Autodesk Inventor part; units mm, degrees
ref_plane "YZ Plane" through (0, 0, 0) normal (1, 0, 0) x (0, 1, 0)
ref_plane "XZ Plane" through (0, 0, 0) normal (0, 1, 0) x (-1, 0, 0)
ref_plane "XY Plane" through (0, 0, 0) normal (0, 0, 1) x (1, 0, 0)
sketch "Sketch1" plane through (0, 0, 0) normal (0, 0, 1) x (1, 0, 0)
  circle A0 centre (0, 0) radius 2.032
  circle A1 centre (0, 0) radius 5.08
  line L0 (3.81, 3.3601) -> (3.81, 5.5534)
  line L1 (-3.81, 3.3601) -> (-3.81, 6.2503)
  circle A2 centre (-20.9, 21.2222) radius 2.032
  circle A3 centre (-20.9, 21.2222) radius 5.08
  line L2 (-17.5399, 25.0322) -> (-14.2921, 25.0322)
  line L3 (-17.5399, 17.4122) -> (-14.7055, 17.4122)
  arc A4 (-3.81, 6.2503) -> (-14.7055, 17.4122) centre (-14.0813, 7.1228) ccw
  arc A5 (3.81, 5.5534) -> (-14.2921, 25.0322) centre (-14.2921, 6.8814) ccw
  point P0 (-3.81, 4.8052)
  dimension "d0" = 4.064
  dimension "d1" = 10.16
  dimension "d2" = 7.62
  dimension "d3" = 3.81
  dimension "d4" = 4.064
  dimension "d5" = 10.16
  dimension "d6" = 7.62
  dimension "d7" = 3.81
extrude "Extrusion1" add sketch "Sketch1" along normal blind 3.556
equation "\"d7\" = 0.5 * d6"
properties part number "Push Arm"
Source: CAD feature listing. Evaluate the final solid. Frame: model axes, mm. A direction names the side the tool comes from. Coordinates: 2 decimals unless noted, no trailing zeros. Loops run counter-clockwise (first coordinate to the right, second up) from the corner with the lowest first, then second, coordinate; pieces in that order, holes last. Notation, with made-up numbers: (-31, 38.5) -> (-7, 38.5) arc R17 cw to (-7, 44.5) -> close; hole circle Ø4 at (53.25, 64). An arc over 180 degrees is marked (long way). One line per item, written item: value. Start each with the question number.
Q1. Section query A-A, the plane y = 0. Return the cut outline in (x, z).
Q2. Contact query for flat-ended pins moving along their axis: P1, Ø2, axis at y = 5, z = 1.5, coming from the +X side; P2, Ø2, axis at y = 5.5, z = 3, coming from the -X side; P3, Ø0.9, axis at x = -17, z = 1.5, coming from the -Y side; P4, Ø2.5, axis at x = -20.9, y = 21.22, coming from the +Z side (3 decimals). Output: stop coordinate, or through.
Q3. Mould query, pull axis Y, two halves, no side actions, for faces 1 (the face through (-3.81, 5, 2)), 2 (the face through (-16, 17.412, 2)), 3 (the face through (-4, 14, 0)), 4 (the face through (-21.34, 23.206, 1.753)). Classes: pulls with the +Y half, pulls with the -Y half, needs draft (parallel to the pull), parting line crosses it, or undercut.
Q4. Set-up query: faces 5 (the face through (-6.79, 14.41, 1.75)), 6 (the face through (-4, 14, 3.556)), 7 (the face through (3.81, 4, 2)), 8 (the face through (-16, 25.032, 2)). Return all of +Z, -Z, +X, -X, +Y, -Y with unobstructed straight access to the full face (end or side cutting, diameter ignored); none if empty.
Q5. Line query: line 1 along Y through (x, z) = (-1.5, 2.1); line 2 along Y through (x, z) = (-16.5, 1.4); line 3 along X through (y, z) = (0.5, 2.3). Output: solid intervals per line, ascending.
Q6. Section query B-B, the plane x = -20.9. Return the cut outline in (y, z), and give its area (3 significant figures).
Q7. Section query C-C, the plane z = 0.45. Return the cut outline in (x, y), and give its area (3 significant figures).
Q8. Section query D-D, the plane y = 10.5. Return the cut outline in (x, z).
Results:
1. outline: (-5.08, 0) -> (-2.03, 0) -> (-2.03, 3.56) -> (-5.08, 3.56) -> close; (2.03, 0) -> (5.08, 0) -> (5.08, 3.56) -> (2.03, 3.56) -> close
2. P1: x = 3.84
2. P2: x = -3.81
2. P3: y = 17.41
2. P4: through
3. face 1: undercut
3. face 2: pulls with the -Y half
3. face 3: needs draft
3. face 4: undercut
4. face 5: +Z, -Z
4. face 6: +Z, +X, -X, +Y, -Y
4. face 7: +Z, -Z, +X
4. face 8: +Z, -Z, +X, +Y
5. line 1: -4.85 to -1.37, 1.37 to 19.76
5. line 2: 17.41 to 25.03
5. line 3: -5.06 to -1.97, 1.97 to 5.06
6. outline: (16.14, 0) -> (19.19, 0) -> (19.19, 3.56) -> (16.14, 3.56) -> close; (23.25, 0) -> (26.3, 0) -> (26.3, 3.56) -> (23.25, 3.56) -> close
6. area: 21.7 mm^2
7. outline: (-17.54, 17.41) -> (-14.71, 17.41) arc R10.31 cw to (-3.81, 6.25) -> (-3.81, 3.36) arc R5.08 ccw (long way) to (3.81, 3.36) -> (3.81, 5.55) arc R18.15 ccw to (-14.29, 25.03) -> (-17.54, 25.03) arc R5.08 ccw (long way) to start; hole circle Ø4.06 at (-20.9, 21.22); hole circle Ø4.06 at (0, 0)
7. area: 340 mm^2
8. outline: (-4.34, 0) -> (3.49, 0) -> (3.49, 3.56) -> (-4.34, 3.56) -> close
